from build123d import *

# Parameters (mm, degrees)
SKETCH_2_R      = 15
EXTRUDE_1_DEPTH = 5


with BuildPart() as part:
    # 草圖2 → 填料-伸長1 (new body)
    with BuildSketch(Plane.XY):
        Circle(SKETCH_2_R)
        with BuildLine():
            Line((0, 5), (0, 12.5))
            ThreePointArc((0, 12.5), (1.631577403, 12.393060767), (3.235238064, 12.074072829))
            Line((3.235238064, 12.074072829), (1.294095226, 4.829629131))
            ThreePointArc((1.294095226, 4.829629131), (0.652630961, 4.957224307), (0, 5))
        make_face(mode=Mode.SUBTRACT)
        with BuildLine():
            Line((2.5, 4.330127019), (6.25, 10.825317547))
            ThreePointArc((6.25, 10.825317547), (7.609517863, 9.916916754), (8.838834765, 8.838834765))
            Line((8.838834765, 8.838834765), (3.535533906, 3.535533906))
            ThreePointArc((3.535533906, 3.535533906), (3.043807145, 3.966766701), (2.5, 4.330127019))
        make_face(mode=Mode.SUBTRACT)
        with BuildLine():
            Line((4.330127019, 2.5), (10.825317547, 6.25))
            ThreePointArc((10.825317547, 6.25), (11.548494156, 4.783542905), (12.074072829, 3.235238064))
            Line((12.074072829, 3.235238064), (4.829629131, 1.294095226))
            ThreePointArc((4.829629131, 1.294095226), (4.619397663, 1.913417162), (4.330127019, 2.5))
        make_face(mode=Mode.SUBTRACT)
        with BuildLine():
            Line((5, 0), (12.5, 0))
            ThreePointArc((12.5, 0), (12.393060767, -1.631577403), (12.074072829, -3.235238064))
            Line((12.074072829, -3.235238064), (4.829629131, -1.294095226))
            ThreePointArc((4.829629131, -1.294095226), (4.957224307, -0.652630961), (5, 0))
        make_face(mode=Mode.SUBTRACT)
        with BuildLine():
            Line((4.330127019, -2.5), (10.825317547, -6.25))
            ThreePointArc((10.825317547, -6.25), (9.916916754, -7.609517863), (8.838834765, -8.838834765))
            Line((8.838834765, -8.838834765), (3.535533906, -3.535533906))
            ThreePointArc((3.535533906, -3.535533906), (3.966766701, -3.043807145), (4.330127019, -2.5))
        make_face(mode=Mode.SUBTRACT)
        with BuildLine():
            Line((2.5, -4.330127019), (6.25, -10.825317547))
            ThreePointArc((6.25, -10.825317547), (4.783542905, -11.548494156), (3.235238064, -12.074072829))
            Line((3.235238064, -12.074072829), (1.294095226, -4.829629131))
            ThreePointArc((1.294095226, -4.829629131), (1.913417162, -4.619397663), (2.5, -4.330127019))
        make_face(mode=Mode.SUBTRACT)
        with BuildLine():
            Line((0, -5), (0, -12.5))
            ThreePointArc((0, -12.5), (-1.631577403, -12.393060767), (-3.235238064, -12.074072829))
            Line((-3.235238064, -12.074072829), (-1.294095226, -4.829629131))
            ThreePointArc((-1.294095226, -4.829629131), (-0.652630961, -4.957224307), (0, -5))
        make_face(mode=Mode.SUBTRACT)
        with BuildLine():
            Line((-2.5, -4.330127019), (-6.25, -10.825317547))
            ThreePointArc((-6.25, -10.825317547), (-7.609517863, -9.916916754), (-8.838834765, -8.838834765))
            Line((-8.838834765, -8.838834765), (-3.535533906, -3.535533906))
            ThreePointArc((-3.535533906, -3.535533906), (-3.043807145, -3.966766701), (-2.5, -4.330127019))
        make_face(mode=Mode.SUBTRACT)
        with BuildLine():
            Line((-4.330127019, -2.5), (-10.825317547, -6.25))
            ThreePointArc((-10.825317547, -6.25), (-11.548494156, -4.783542905), (-12.074072829, -3.235238064))
            Line((-12.074072829, -3.235238064), (-4.829629131, -1.294095226))
            ThreePointArc((-4.829629131, -1.294095226), (-4.619397663, -1.913417162), (-4.330127019, -2.5))
        make_face(mode=Mode.SUBTRACT)
        with BuildLine():
            Line((-5, 0), (-12.5, 0))
            ThreePointArc((-12.5, 0), (-12.393060767, 1.631577403), (-12.074072829, 3.235238064))
            Line((-12.074072829, 3.235238064), (-4.829629131, 1.294095226))
            ThreePointArc((-4.829629131, 1.294095226), (-4.957224307, 0.652630961), (-5, 0))
        make_face(mode=Mode.SUBTRACT)
        with BuildLine():
            Line((-4.330127019, 2.5), (-10.825317547, 6.25))
            ThreePointArc((-10.825317547, 6.25), (-9.916916754, 7.609517863), (-8.838834765, 8.838834765))
            Line((-8.838834765, 8.838834765), (-3.535533906, 3.535533906))
            ThreePointArc((-3.535533906, 3.535533906), (-3.966766701, 3.043807145), (-4.330127019, 2.5))
        make_face(mode=Mode.SUBTRACT)
        with BuildLine():
            Line((-2.5, 4.330127019), (-6.25, 10.825317547))
            ThreePointArc((-6.25, 10.825317547), (-4.783542905, 11.548494156), (-3.235238064, 12.074072829))
            Line((-3.235238064, 12.074072829), (-1.294095226, 4.829629131))
            ThreePointArc((-1.294095226, 4.829629131), (-1.913417162, 4.619397663), (-2.5, 4.330127019))
        make_face(mode=Mode.SUBTRACT)
        with BuildLine():
            Line((1, -1.118033989), (1, 1.118033989))
            ThreePointArc((1, 1.118033989), (-1.5, 0), (1, -1.118033989))
        make_face(mode=Mode.SUBTRACT)
    extrude(amount=EXTRUDE_1_DEPTH)


solid = part.part
Check sheet for the modelled part. Datum: model origin and axes. Units: mm. Round coordinates to 2 decimals unless told otherwise and drop trailing zeros. Loops run counter-clockwise (first coordinate to the right, second up) from the corner with the lowest first, then second, coordinate; pieces in that order, holes last. Notation, with made-up numbers: M 24,68 L 62,68 A24 ccw 62,105 Z; hole C -37,-12 d3. An arc over 180 degrees is marked long. One line per item, written item: value.
(1) Depth check by flat-ended pin: pin 1 Ø2 at (x, z) = (4.5, 4) entering from +Y; pin 2 Ø2.5 at (y, z) = (8.5, 1.5) entering from +X; pin 3 Ø2.5 at (x, z) = (-10, 3.5) entering from +Y. Enter the tip coordinate at first touch or a pass-through.
Computed values:
pin 1: stops at y = 14.59
pin 2: stops at x = 13.13
pin 3: stops at y = 12.18
(2) Release check for a two-part mould opening along Y. For faces 1 (the face through (9.93, -7.59, 2.46)), 2 (the face through (-4.623, -1.905, 2.465)) record: +Y half, -Y half, draft (parallel to the pull), parting line (faces both ways), or undercut.
Computed values:
face 1: undercut
face 2: undercut
(3) Sectioned sample at B-B, the plane z = 4.1. Count the separate pieces of the cut face and the enclosed holes in it, then the cut area to 3 significant figures.
Computed values:
separate pieces: 1
enclosed holes: 13
area: 494 mm^2
(4) Sectioned sample at A-A, the plane x = 10.25. Record the cut outline in (y, z).
Computed values:
outline: M -10.95,0 L -7.15,0 L -7.15,5 L -10.95,5 Z; M -5.92,0 L -2.75,0 L -2.75,5 L -5.92,5 Z; M 0,0 L 2.75,0 L 2.75,5 L 0,5 Z; M 5.92,0 L 10.95,0 L 10.95,5 L 5.92,5 Z
(5) Sectioned sample at C-C, the plane y = 11.5. Record the cut outline in (x, z), then the cut area to 3 significant figures.
Computed values:
outline: M -9.63,0 L -4.9,0 L -4.9,5 L -9.63,5 Z; M -3.08,0 L 0,0 L 0,5 L -3.08,5 Z; M 3.08,0 L 9.63,0 L 9.63,5 L 3.08,5 Z
area: 71.8 mm^2
(6) Thickness scan on line 1 (X direction, y = -9, z = 4); line 2 (Y direction, x = -11, z = 1.5); line 3 (X direction, y = -0.75, z = 2.5). Record the ranges inside material, lowest first.
Computed values:
line 1: x = -12 to -8.67, -5.2 to -2.41, 0 to 2.41, 5.2 to 12
line 2: y = -10.2 to -5.94, -2.95 to 0, 2.95 to 10.2
line 3: x = -14.98 to -1.3, 1 to 4.94, 12.48 to 14.98
